Can you work these out from the model? Positions are in its coordinate system, mm. A direction names the side the tool comes from. Coordinates: 2 decimals unless noted, no trailing zeros. Loops run counter-clockwise (first coordinate to the right, second up) from the corner with the lowest first, then second, coordinate; pieces in that order, holes last. Notation, with made-up numbers: (-7, -2) - (32, -2) arc R19 ccw to (32, 30) - close; hole circle Ø9 at (-37.5, -9). An arc over 180 degrees is marked (long way). Put each result on its own line as item: value. Start each with the question number.
Autodesk Inventor part; units mm, degrees
ref_plane "YZ Plane" through (0, 0, 0) normal (1, 0, 0) x (0, 1, 0)
ref_plane "XZ Plane" through (0, 0, 0) normal (0, 1, 0) x (-1, 0, 0)
ref_plane "XY Plane" through (0, 0, 0) normal (0, 0, 1) x (1, 0, 0)
sketch "Sketch1" plane through (0, 0, 0) normal (0, 1, 0) x (-1, 0, 0)
  line L0 (-8.0312, -19.6194) -> (-8.0312, -0.5694)
  line L1 (-8.0312, -0.5694) -> (-34.5277, -0.5694)
  line L2 (-34.5277, -0.5694) -> (-34.5277, -28.5056)
  line L3 (18.6455, 5.0782) -> (18.6456, 5.0782)
  line L4 (-1.974, -37.6808) -> (-8.0312, -19.6194)
  line L5 (-34.5277, -28.5056) -> (-27.4611, -49.5771)
  line L6 (-1.974, -37.6808) -> (-0.9645, -40.691)
  line L7 (-27.4611, -49.5771) -> (-0.9645, -40.691)
  circle A0 centre (-21.2794, -10.0945) radius 2.4447
  line L8 (-8.0312, -0.5694) -> (-8.0312, -19.6194)
  line L9 (-8.0312, -19.6194) -> (-0.9645, -40.691)
  line L10 (-0.9645, -40.691) -> (-27.4611, -49.5771)
  line L11 (-27.4611, -49.5771) -> (-34.5277, -28.5056)
  line L12 (-34.5277, -28.5056) -> (-34.5277, -0.5694)
  line L13 (-34.5277, -0.5694) -> (-8.0312, -0.5694)
  dimension "d0" = 19.05
  dimension "d1" = 22.225
  dimension "d2" = 27.9469
  dimension "d3" = 26.4965
  dimension "d4" = 4.8895
  dimension "d18" = 13.2483
  dimension "d19" = 9.525
  dimension "d20" = 161.46
extrude "Extrusion1" add sketch "Sketch1" along normal blind 5.6134
sketch "Sketch2" plane through (0, 0, 0) normal (0, -1, 0) x (1, 0, 0)
  line L0 (27.4611, -49.5771) -> (0.9645, -40.691)
  line L1 (31.5175, -27.4959) -> (29.9883, -26.9832)
  line L2 (34.5277, -28.5056) -> (27.4611, -49.5771)
  line L3 (27.4611, -49.5771) -> (0.9645, -40.691)
  line L4 (31.5175, -27.4959) -> (8.0312, -19.6194)
  line L5 (8.0312, -19.6194) -> (7.0136, -22.6537)
  line L6 (7.0136, -22.6537) -> (27.4656, -29.5126)
  line L7 (24.4508, -48.5675) -> (21.4165, -47.5499)
  line L8 (21.4165, -47.5499) -> (27.4656, -29.5126)
  line L9 (29.9883, -26.9831) -> (31.5175, -27.4959)
  line L10 (31.5175, -27.4959) -> (24.4508, -48.5675)
  point P0 (0, 0)
  dimension "d15" = 3.2004
  dimension "d16" = 3.175
  dimension "d17" = 3.2004
extrude "Extrusion2" cut sketch "Sketch2" against normal blind 1.5875
fillet "Fillet1" radius 1.5875 1 edges at (31.5175, 0.7937, -27.4959)
properties part number "Lidar Sensor CAse Piece 1"
Q1. Please list where these lines run through material, in increasing order: line 1 along X through (y, z) = (1.45, -4.5); line 2 along X through (y, z) = (3.9, -8); line 3 along X through (y, z) = (3.95, -8.5). Write a range as [from, to].
Q2. We'd pull the mould along X, two halves only. Please class faces 1 (the flat face through (18, 5.613, -25)), 2 (the flat face through (31.044, 2.767, -38.894)), 3 (the cylindrical face through (18.95, 2.77, -10.83)): released by +X, released by -X, zero draft, split by the parting line, or undercut.
Q3. I want a section at D-D on x = 9.5. List the corners of the cut face in (y, z) for me.
Q4. I want a section at C-C on z = -15. List the corners of the cut face in (x, y) for me.
Q5. I want a section at B-B on x = 29.5. List the corners of the cut face in (y, z) for me.
Q6. I want a section at A-A on y = 0.9. Count the separate pieces of the cut face and the enclosed holes in it, and give its area (3 significant figures).
Q7. On a 3-axis mill with a long thin cutter (end or side, diameter ignored), from which of +Z, -Z, +X, -X, +Y, -Y can I reach the whole of each face in a straight line? I mean faces 4 (the flat face through (8.031, 3, -10)), 5 (the flat face through (17.096, 0.783, -26.035)), 6 (the flat face through (14, 0, -35)). Say none if no direction works.
Calculated:
1. line 1: [8.03, 34.53]
1. line 2: [8.03, 20.02], [22.54, 34.53]
1. line 3: [8.03, 19.43], [23.13, 34.53]
2. face 1: zero draft
2. face 2: released by +X
2. face 3: undercut
3. outline: (0, -43.55) - (5.61, -43.55) - (5.61, -0.57) - (0, -0.57) - (0, -20.11) - (1.59, -20.11) - (1.59, -23.49) - (0, -23.49) - close
4. outline: (8.03, 0) - (34.53, 0) - (34.53, 5.61) - (8.03, 5.61) - close
5. outline: (0, -43.5) - (5.61, -43.5) - (5.61, -0.57) - (0, -0.57) - (0, -26.82) - (1.59, -26.82) - (1.59, -33.51) - (0, -33.51) - close
6. separate pieces: 2
6. enclosed holes: 1
6. area: 1,090 mm2
7. face 4: +Z, -X, +Y, -Y
7. face 5: -Y
7. face 6: +Z, -Z, +X, -X, -Y
